Could you check a few things on this model? Use its own coordinates, in mm. Coordinates: 2 decimals unless noted, no trailing zeros. Loops run counter-clockwise (first coordinate to the right, second up) from the corner with the lowest first, then second, coordinate; pieces in that order, holes last. Notation, with made-up numbers: (72, 74.5) - (100, 74.5) arc R9 ccw to (100, 80.5) - close; hole circle Ø8 at (80, 72). An arc over 180 degrees is marked (long way). One line per question, with ' | ' between items. Start each with the question number.
1. I want a section at A-A, the plane z = 3.5. Write out the boundary of the cut face in (x, y) (3 decimals), then the cut area to 3 significant figures.
2. I want a section at C-C, the plane y = -603.5. Write out the boundary of the cut face in (x, z), then the cut area to 3 significant figures.
3. I want a section at B-B, the plane x = 80. Write out the boundary of the cut face in (y, z).
4. Please list where these lines run through material, in increasing order: L1, parallel to X at y = -153.5, z = 3.75; L2, parallel to X at y = -166, z = 2.5; L3, parallel to X at y = -427, z = 1.75. Write a range as [from, to].
from build123d import *

# Parameters (mm, degrees)
F1_DEPTH = 6.35


with BuildPart() as f1:
    # F0 (on Top) → F1 (new body)
    with BuildSketch(Plane.XY):
        Polygon((101.6, 0), (0, 0), (0, -736.6), (50.8, -736.6), (101.6, -127), align=None)
        with BuildLine():
            ThreePointArc((19.05, -133.35), (22.225, -130.175), (25.4, -133.35))
            Line((25.4, -133.35), (25.4, -165.1))
            ThreePointArc((25.4, -165.1), (22.225, -168.275), (19.05, -165.1))
            Line((19.05, -165.1), (19.05, -133.35))
        make_face(mode=Mode.SUBTRACT)
    extrude(amount=F1_DEPTH)


solid = f1.part
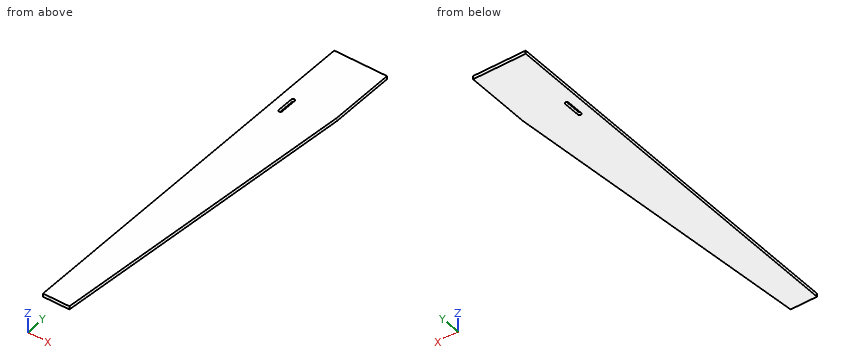
Results are:
1) outline: (0, -736.6) - (50.8, -736.6) - (101.6, -127) - (101.6, 0) - (0, 0) - close; hole (19.05, -165.1) arc R3.175 ccw to (25.4, -165.1) - (25.4, -133.35) arc R3.175 ccw to (19.05, -133.35) - close | area: 59,100 mm2
2) outline: (0, 0) - (61.89, 0) - (61.89, 6.35) - (0, 6.35) - close | area: 393 mm2
3) outline: (-386.2, 0) - (0, 0) - (0, 6.35) - (-386.2, 6.35) - close
4) L1: x = [0, 19.05], [25.4, 99.39] | L2: x = [0, 19.18], [25.27, 98.35] | L3: x = [0, 76.6]
